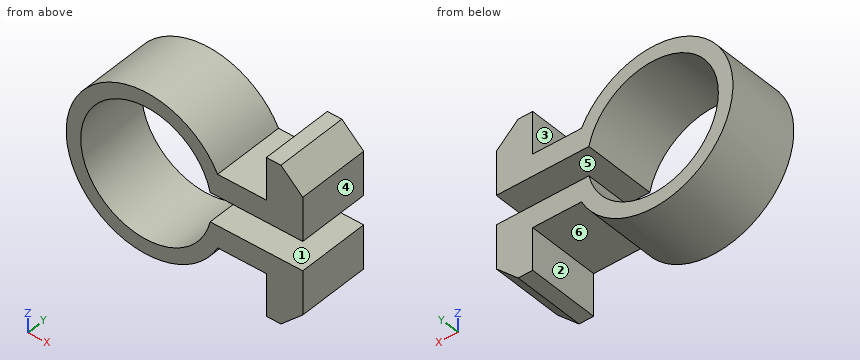
Autodesk Inventor part; units mm, degrees
ref_plane "YZ Plane" through (0, 0, 0) normal (1, 0, 0) x (0, 1, 0)
ref_plane "XZ Plane" through (0, 0, 0) normal (0, 1, 0) x (-1, 0, 0)
ref_plane "XY Plane" through (0, 0, 0) normal (0, 0, 1) x (1, 0, 0)
sketch "Sketch1" plane through (0, 0, 0) normal (0, 1, 0) x (-1, 0, 0)
  arc A0 (-4.3875, -1) -> (-4.3875, 1) centre (0, 0) ccw
  line L0 (-10.75, -1) -> (-4.3875, -1)
  line L1 (-8.25, -2.5) -> (-4.899, -2.5)
  line L2 (0, 0) -> (18.2262, 0) construction
  line L3 (-8.25, -2.5) -> (-8.25, -5.4)
  line L4 (-10.75, -1) -> (-10.75, -4)
  line L5 (-8.25, -5.4) -> (-9.25, -5.4)
  line L6 (-9.25, -5.4) -> (-10.75, -4)
  line L7 (-10.75, 1) -> (-4.3875, 1)
  line L8 (-8.25, 2.5) -> (-4.899, 2.5)
  line L9 (-8.25, 2.5) -> (-8.25, 5.4)
  line L10 (-10.75, 1) -> (-10.75, 4)
  line L11 (-8.25, 5.4) -> (-9.25, 5.4)
  line L12 (-9.25, 5.4) -> (-10.75, 4)
  arc A1 (-4.899, -2.5) -> (-4.899, 2.5) centre (0, 0) ccw
  point P0 (-5.692, 1)
  dimension "d0" = 9
  dimension "d3" = 1.5
  dimension "d4" = 1
  dimension "d7" = 3
  dimension "d10" = 4.4
  dimension "d16" = 1
  dimension "d17" = 3.351
  dimension "d18" = 5.5
  dimension "d20" = 2.5
extrude "Extrusion1" add sketch "Sketch1" along normal blind 5
properties part number "V Slot Clip Wire Holder"
Can you work these out from the model? Positions are in its coordinate system, mm. Face numbers are marked on the shaded views. A direction names the side the tool comes from. Give positions to 0.01 mm unless a question says otherwise; leave off trailing zeros. Loops run counter-clockwise (first coordinate to the right, second up) from the corner with the lowest first, then second, coordinate; pieces in that order, holes last. Notation, with made-up numbers: M -11,26 L 42,26 A16 cw 42,33 Z; hole C 11.25,-4 d9. An arc over 180 degrees is marked long. One line per item, written item: value.
(1) Suppose I cut it at B-B on y = 3.85. List the corners of the cut face in (x, z) for me.
Returned:
outline: M 4.39,-1 A4.5 cw long 4.39,1 L 10.75,1 L 10.75,4 L 9.25,5.4 L 8.25,5.4 L 8.25,2.5 L 4.9,2.5 A5.5 ccw long 4.9,-2.5 L 8.25,-2.5 L 8.25,-5.4 L 9.25,-5.4 L 10.75,-4 L 10.75,-1 Z
(2) We'd pull the mould along Z, two halves only. Please class the marked faces 4, 5 and 6: released by +Z, released by -Z, zero draft, split by the parting line, or undercut.
Returned:
face 4: zero draft
face 5: undercut
face 6: released by -Z
(3) Suppose I cut it at A-A on x = 0. List the corners of the cut face in (y, z) for me, plus the area to 3 significant figures.
Returned:
outline: M 0,-5.5 L 5,-5.5 L 5,-4.5 L 0,-4.5 Z; M 0,4.5 L 5,4.5 L 5,5.5 L 0,5.5 Z
area: 10.0 mm^2
(4) Will these pins go through, and if not, where does the flat tip stop? pin 1 (3 mm diameter, centred on y = 1.5, z = -4, fed in from -X); pin 2 (1.5 mm diameter, centred on y = 3.5, z = -4, fed in from -X); pin 3 (0.8 mm diameter, centred on x = 9, y = 3.5, fed in from -Z).
Returned:
pin 1: x = -4.9
pin 2: x = -4.44
pin 3: z = -5.4
(5) Suppose I cut it at C-C on z = -1.5. List the corners of the cut face in (x, y) for me, plus the area to 3 significant figures.
Returned:
outline: M -5.29,0 L -4.24,0 L -4.24,5 L -5.29,5 Z; M 4.24,0 L 10.75,0 L 10.75,5 L 4.24,5 Z
area: 37.8 mm^2
(6) I need wall thicknesses on line 1 (Z direction, x = 0, y = 2.9); line 2 (Z direction, x = 5.75, y = 2.6); line 3 (X direction, y = 0.4, z = -3). Which ranges of each line are inside material? Lowest first, please.
Returned:
line 1: -5.5 to -4.5, 4.5 to 5.5
line 2: -2.5 to -1, 1 to 2.5
line 3: -4.61 to -3.35, 3.35 to 4.61, 8.25 to 10.75
(7) Suppose I cut it at D-D on z = 0. List the corners of the cut face in (x, y) for me.
Returned:
outline: M -5.5,0 L -4.5,0 L -4.5,5 L -5.5,5 Z
(8) Which directions (+Z, -Z, +X, -X, +Y, -Y) give clear straight access to the entire face, cutting with the end or side of a thin tool? Please do the marked faces 1, 2 and 3.
Returned:
face 1: +X, +Y, -Y
face 2: -Z, +Y, -Y
face 3: +Z, +Y, -Y
